Input: dimensioned drawing with shaded views. Units: mm. Origin: part minimum x, y, z. A direction names the side the tool comes from. Round coordinates to 2 decimals unless told otherwise and drop trailing zeros. Order: outer loops, then holes, each group sorted by start corner. A loop starts at its lowest first (then second) coordinate and runs counter-clockwise, first axis right, second up. Notation, with made-up numbers: (16.25, 43.25) - (68.25, 43.25) arc R23 ccw to (68.25, 65.25) - close; hole circle Ø4 at (28, 26). An arc over 180 degrees is marked (long way). Return JSON: item names as keys, results as strings. Group by question number.
1) Section B-B, the plane x = 10. Return loops of the section in (y, z).
2) Section D-D, the plane x = 112.5. Return loops of the section in (y, z), plus the area to 3 significant figures.
3) Mould query, pull axis Y, two halves, no side actions, for the marked faces 1, 2, 3 and 4. Classes: pulls with the +Y half, pulls with the -Y half, needs draft (parallel to the pull), parting line crosses it, or undercut.
4) Ray query, line 1 (Z direction, x = 75, y = 56.5); line 2 (X direction, y = 74, z = 30). Return the intervals inside material, ascending. Write a range as from..to.
5) Section C-C, the plane y = 43. Return loops of the section in (x, z).
6) Access query for the marked faces 5, 6 and 7. Directions: +Z, -Z, +X, -X, +Y, -Y. A direction counts if a zero-diameter tool reaches every point of the face in a straight line with its end or side. Return the directions, or none.
7) Contact query for flat-ended pins moving along their axis: P1, Ø8, axis at x = 13, y = 16.5, coming from the -Z side; P2, Ø2, axis at x = 55.5, y = 44, coming from the -Z side. Output: stop coordinate, or through.
8) Section A-A, the plane z = 34. Return loops of the section in (x, y), plus the area to 3 significant figures.
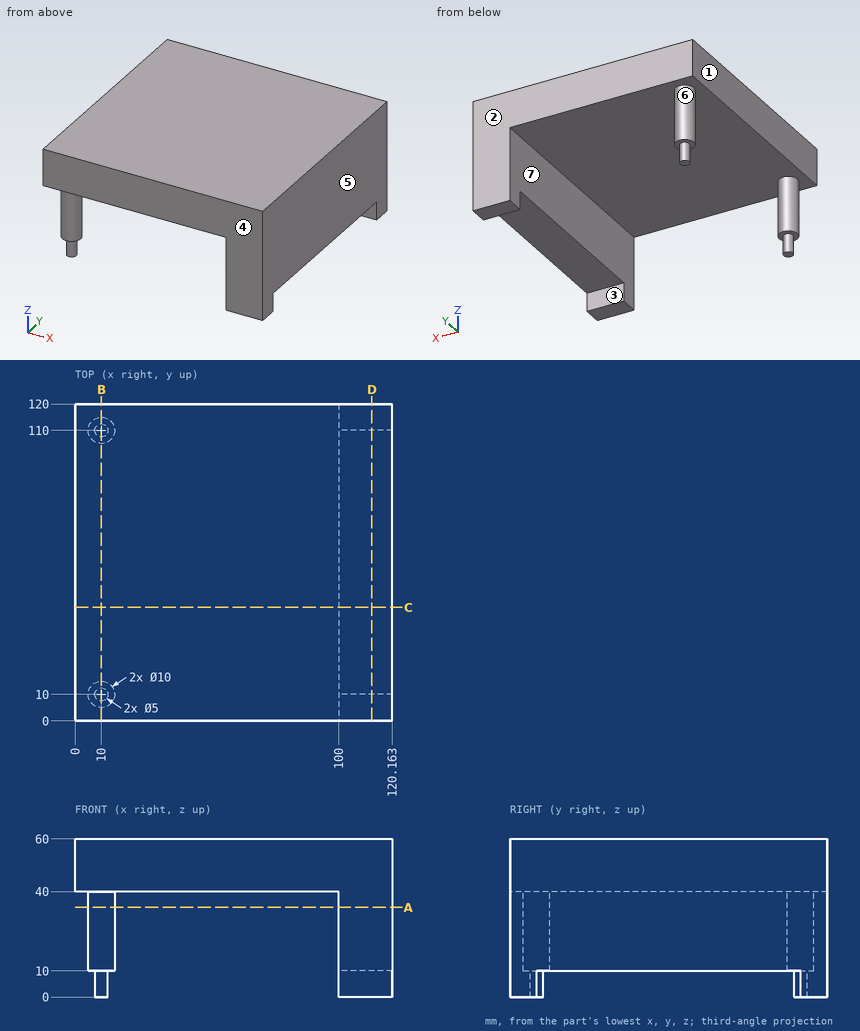
Geometry check:
{
 "1": {"outline": "(0, 40) - (5, 40) - (5, 10) - (7.5, 10) - (7.5, 0) - (12.5, 0) - (12.5, 10) - (15, 10) - (15, 40) - (105, 40) - (105, 10) - (107.5, 10) - (107.5, 0) - (112.5, 0) - (112.5, 10) - (115, 10) - (115, 40) - (120, 40) - (120, 60) - (0, 60) - close"},
 "2": {"outline": "(0, 0) - (10, 0) - (10, 10) - (110, 10) - (110, 0) - (120, 0) - (120, 60) - (0, 60) - close", "area": "6,200 mm2"},
 "3": {"face 1": "needs draft", "face 2": "pulls with the +Y half", "face 3": "undercut", "face 4": "pulls with the -Y half"},
 "4": {"line 1": "40..60", "line 2": "100..120.16"},
 "5": {"outline": "(0, 40) - (100, 40) - (100, 10) - (120.16, 10) - (120.16, 60) - (0, 60) - close"},
 "6": {"face 5": "+Z, -Z, +X, +Y, -Y", "face 6": "-Z", "face 7": "-Z, +Y, -Y"},
 "7": {"P1": "z = 10", "P2": "z = 40"},
 "8": {"outline": "circle Ø10 at (10, 10); circle Ø10 at (10, 110); (100, 0) - (120.16, 0) - (120.16, 120) - (100, 120) - close", "area": "2,580 mm2"}
}
